Here's how the part is built. I have some questions about the finished solid (model axes, mm). Round coordinates to 2 decimals unless told otherwise and drop trailing zeros. Loops run counter-clockwise (first coordinate to the right, second up) from the corner with the lowest first, then second, coordinate; pieces in that order, holes last. Notation, with made-up numbers: (-25.75, 23.25) -> (10.25, 23.25) arc R27 ccw to (10.25, 60.25) -> close; hole circle Ø3 at (27, 29). An arc over 180 degrees is marked (long way). Use one line per item in the form item = value. Start each with the question number.
Item 1: If we section it at B-B (y = 3.75): Write out the boundary of the cut face in (x, z), then the cut area to 3 significant figures.
Item 2: I'm going to push flat-ended pins straight in: pin 1 Ø4 at (x, z) = (7, 17.5) entering from -Y; pin 2 Ø6 at (x, z) = (10, 9) entering from +Y; pin 3 Ø1.5 at (x, z) = (9.5, 20.5) entering from +Y. Where does each tip first touch, or does it pass through?
Item 3: If we section it at C-C (z = 23.75): Write out the boundary of the cut face in (x, y).
Item 4: If I drill on L1, parallel to Z at x = 8, y = 24.75; L2, parallel to Y at x = 5.5, z = 17; L3, parallel to Y at x = 23.25, z = 19.25, over which ranges is the centre line in solid material (lowest first)? Write a range as [from, to].
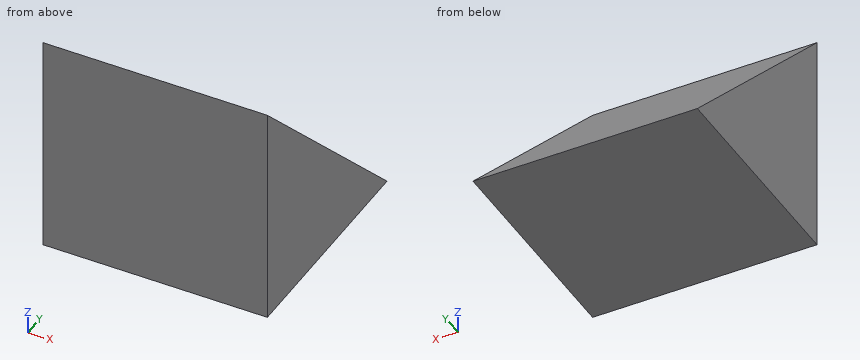
Autodesk Inventor part; units mm, degrees
ref_plane "YZ Plane" through (0, 0, 0) normal (1, 0, 0) x (0, 1, 0)
ref_plane "XZ Plane" through (0, 0, 0) normal (0, 1, 0) x (-1, 0, 0)
ref_plane "XY Plane" through (0, 0, 0) normal (0, 0, 1) x (1, 0, 0)
sketch "Sketch1" plane through (0, 0, 0) normal (1, 0, 0) x (0, 1, 0)
  line L0 (0, 0) -> (30, 0)
  line L1 (30, 0) -> (30, 30)
  line L2 (30, 30) -> (0, 30)
  line L3 (0, 30) -> (0, 0)
  dimension "d0" = 30
  dimension "d1" = 30
extrude "Extrusion1" add sketch "Sketch1" along normal blind 30
chamfer "Chamfer1" distance 30 angle 45 1 edges at (15, 30, 30)
properties part number "edge"
Values found:
q1.outline = (0, 0) -> (30, 0) -> (30, 26.25) -> (0, 26.25) -> close
q1.area = 788 mm2
q2.pin_1 = 0
q2.pin_2 = 24
q2.pin_3 = 10.25
q3.outline = (0, 0) -> (30, 0) -> (30, 6.25) -> (0, 6.25) -> close
q4.L1 = [0, 5.25]
q4.L2 = [0, 13]
q4.L3 = [0, 10.75]
